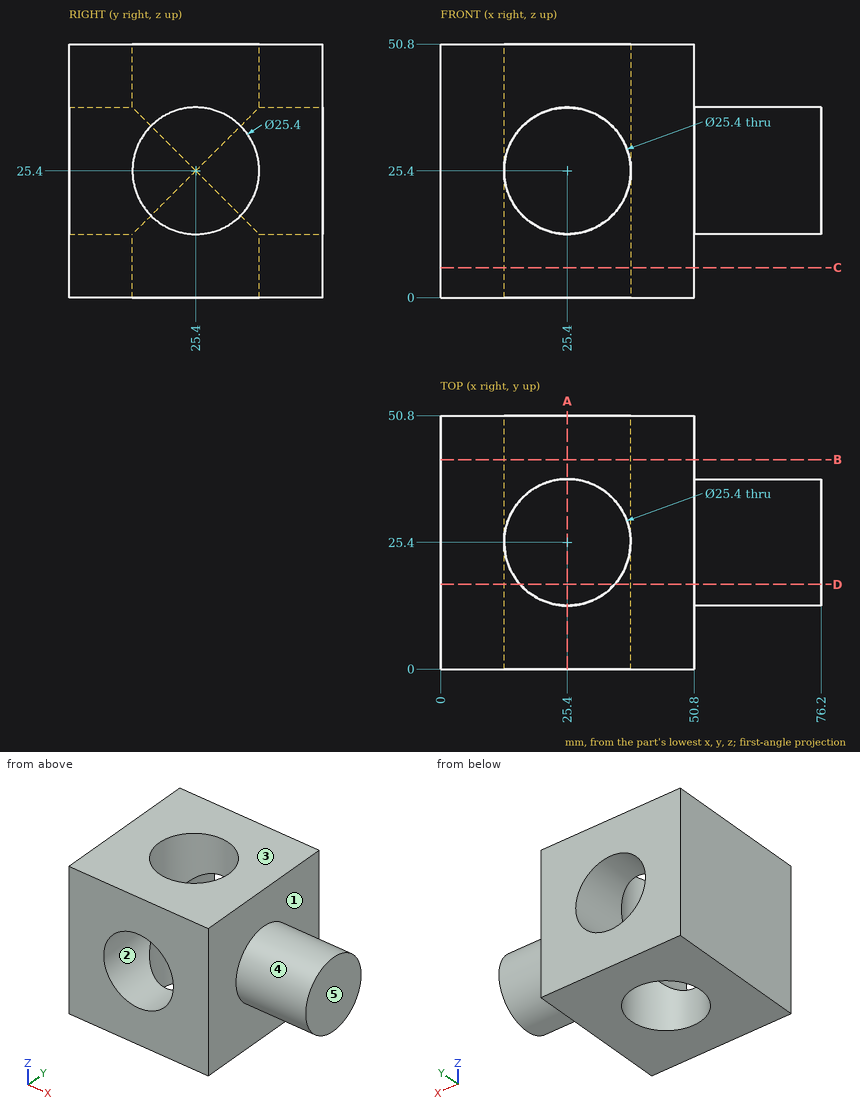
Input: dimensioned drawing with shaded views. Units: mm. Origin: part minimum x, y, z. A direction names the side the tool comes from. Coordinates: 2 decimals unless noted, no trailing zeros. Loops run counter-clockwise (first coordinate to the right, second up) from the corner with the lowest first, then second, coordinate; pieces in that order, holes last. Notation, with made-up numbers: (57, 78.5) -> (87, 78.5) arc R19 cw to (87, 112.5) -> close; hole circle Ø1 at (-34.5, 25.25). An arc over 180 degrees is marked (long way). One line per item, written item: value. Start each with the question number.
Q1. Set-up query: the marked faces 4 and 5. Return all of +Z, -Z, +X, -X, +Y, -Y with unobstructed straight access to the full face (end or side cutting, diameter ignored); none if empty.
Q2. Section query B-B, the plane y = 42. Return the cut outline in (x, z).
Q3. Mould query, pull axis Z, two halves, no side actions, for the marked faces 1, 2 and 3. Classes: pulls with the +Z half, pulls with the -Z half, needs draft (parallel to the pull), parting line crosses it, or undercut.
Q4. Line query: line 1 along Z through (x, y) = (26, 12.5); line 2 along Y through (x, z) = (25.4, 42.5); line 3 along X through (y, z) = (44, 4.5). Output: solid intervals per line, ascending.
Q5. Contact query for flat-ended pins moving along their axis: P1, Ø23, axis at x = 25.4, y = 25.4, coming from the -Z side; P2, Ø1, axis at y = 19, z = 44.5, coming from the +X side; P3, Ø1.5, axis at x = 58.5, y = 17.5, coming from the +Z side. Output: stop coordinate, or through.
Q6. Section query D-D, the plane y = 17. Return the cut outline in (x, z), and give its area (3 significant figures).
Q7. Section query A-A, the plane x = 25.4. Return the cut outline in (y, z).
Results:
1. face 4: +X
1. face 5: +Z, -Z, +X, +Y, -Y
2. outline: (0, 0) -> (50.8, 0) -> (50.8, 50.8) -> (0, 50.8) -> close; hole circle Ø25.4 at (25.4, 25.4)
3. face 1: needs draft
3. face 2: undercut
3. face 3: pulls with the +Z half
4. line 1: 0 to 12.71, 38.09 to 50.8
4. line 2: 0 to 12.7, 38.1 to 50.8
4. line 3: 0 to 50.8
5. P1: through
5. P2: x = 50.8
5. P3: z = 35.9
6. outline: (0, 0) -> (15.87, 0) -> (15.87, 17) arc R12.7 cw to (15.87, 33.8) -> (15.87, 50.8) -> (0, 50.8) -> close; (34.93, 0) -> (50.8, 0) -> (50.8, 15.87) -> (76.2, 15.87) -> (76.2, 34.93) -> (50.8, 34.93) -> (50.8, 50.8) -> (34.93, 50.8) -> (34.93, 33.8) arc R12.7 cw to (34.93, 17) -> close
6. area: 2,020 mm^2
7. outline: (0, 0) -> (12.7, 0) -> (12.7, 12.7) -> (0, 12.7) -> close; (0, 38.1) -> (12.7, 38.1) -> (12.7, 50.8) -> (0, 50.8) -> close; (38.1, 0) -> (50.8, 0) -> (50.8, 12.7) -> (38.1, 12.7) -> close; (38.1, 38.1) -> (50.8, 38.1) -> (50.8, 50.8) -> (38.1, 50.8) -> close
